Here's how the part is built. I have some questions about the finished solid (model axes, mm). Face numbers are marked on the shaded views. A direction names the side the tool comes from. Round coordinates to 2 decimals unless told otherwise and drop trailing zeros. Order: outer loops, then holes, each group sorted by start corner. A loop starts at its lowest first (then second) coordinate and runs counter-clockwise, first axis right, second up.
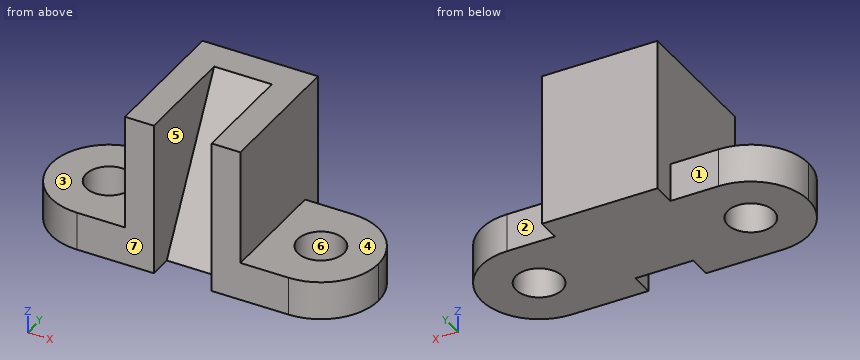
```python
from build123d import *

# Parameters (mm, degrees)
EXTRUDE_1_DEPTH     = 10
SKETCH_3_W          = 30
SKETCH_3_H          = 36
EXTRUDE_2_DEPTH     = 30
SKETCH_4_R          = 6
CUT_EXTRUDE_1_DEPTH = 52
CUT_EXTRUDE_START   = -7.5
CUT_EXTRUDE_2_DEPTH = 15


with BuildPart() as part:
    # 草图1 → 凸台-拉伸1 (new body)
    with BuildSketch(Plane.XY):
        with BuildLine():
            Line((15, -18), (-15, -18))
            Line((-15, -18), (-27.5, -18))
            ThreePointArc((-27.5, -18), (-38.106601718, -13.606601718), (-42.5, -3))
            ThreePointArc((-42.5, -3), (-38.106601718, 7.606601718), (-27.5, 12))
            Line((-27.5, 12), (-15, 12))
            Line((-15, 12), (-15, 18))
            Line((-15, 18), (15, 18))
            Line((15, 18), (15, 12))
            Line((15, 12), (27.5, 12))
            ThreePointArc((27.5, 12), (38.106601718, 7.606601718), (42.5, -3))
            ThreePointArc((42.5, -3), (38.106601718, -13.606601718), (27.5, -18))
            Line((27.5, -18), (15, -18))
        make_face()
    extrude(amount=EXTRUDE_1_DEPTH)

    # 草图3 → 凸台-拉伸2 (add)
    with BuildSketch(Plane.XY.offset(10)):
        Rectangle(SKETCH_3_W, SKETCH_3_H)
    extrude(amount=EXTRUDE_2_DEPTH)

    # 草图4 → 切除-拉伸1 (cut)
    with BuildSketch(Plane.XY):
        with Locations(Location((-27.5, -3, 0), (0, 0, 180))):
            Circle(SKETCH_4_R)
        with Locations(Location((27.511001478, -3, 0), (0, 0, 180))):
            Circle(SKETCH_4_R)
    extrude(amount=CUT_EXTRUDE_1_DEPTH, mode=Mode.SUBTRACT)

    # 草图5 → 切除-拉伸2 (cut)
    with BuildSketch(Plane.ZY.offset(15).offset(CUT_EXTRUDE_START)):
        Polygon((40, 10), (0, -12), (0, -18), (40, -18), align=None)
    extrude(amount=-CUT_EXTRUDE_2_DEPTH, mode=Mode.SUBTRACT)


solid = part.part
```
1. If we section it at D-D, the plane z = 28: Write out the boundary of the cut face in (x, y), and give its area (3 significant figures).
Evaluation:
outline: (-15, -18) - (-7.5, -18) - (-7.5, 3.4) - (7.5, 3.4) - (7.5, -18) - (15, -18) - (15, 18) - (-15, 18) - close
area: 759 mm2
2. If we section it at C-C, the plane z = 3: Write out the boundary of the cut face in (x, y), and give its area (3 significant figures).
Evaluation:
outline: (-27.5, -18) - (-7.5, -18) - (-7.5, -10.35) - (7.5, -10.35) - (7.5, -18) - (27.5, -18) arc R15 ccw to (27.5, 12) - (15, 12) - (15, 18) - (-15, 18) - (-15, 12) - (-27.5, 12) arc R15 ccw to start; hole circle Ø12 at (-27.5, -3); hole circle Ø12 at (27.51, -3)
area: 2,200 mm2
3. I'm going to push flat-ended pins straight in: P1, Ø12, axis at y = 12, z = 26, coming from the +X side; P2, Ø8.5, axis at y = 1, z = 20.5, coming from the -X side; P3, Ø11, axis at x = -21, z = 5, coming from the +Y side. Where does each tip first touch, or does it pass through?
Evaluation:
P1: stops at x = 15
P2: stops at x = -15
P3: stops at y = 12
4. If we section it at A-A, the plane y = -15: Write out the boundary of the cut face in (x, z), and give its area (3 significant figures).
Evaluation:
outline: (-36.5, 0) - (-7.5, 0) - (-7.5, 40) - (-15, 40) - (-15, 10) - (-36.5, 10) - close; (7.5, 0) - (36.5, 0) - (36.5, 10) - (15, 10) - (15, 40) - (7.5, 40) - close
area: 1,030 mm2
5. I need wall thicknesses on probe 1 along Y at (x, z) = (-27.5, 2.25); probe 2 along X at (y, z) = (2, 38); probe 3 along Z at (x, y) = (36, -2). Which ranges of each line are inside material? Lowest first, please.
Evaluation:
probe 1: y = -18 to -9, 3 to 12
probe 2: x = -15 to -7.5, 7.5 to 15
probe 3: z = 0 to 10
6. If we section it at B-B, the plane y = 1: Write out the boundary of the cut face in (x, z).
Evaluation:
outline: (-41.96, 0) - (-31.97, 0) - (-31.97, 10) - (-41.96, 10) - close; (-23.03, 0) - (23.04, 0) - (23.04, 10) - (15, 10) - (15, 40) - (7.5, 40) - (7.5, 23.64) - (-7.5, 23.64) - (-7.5, 40) - (-15, 40) - (-15, 10) - (-23.03, 10) - close; (31.98, 0) - (41.96, 0) - (41.96, 10) - (31.98, 10) - close
7. If we mould it in two halves opening along X, with no side actions, what happens to the marked faces 6 and 7? For each: released by +X, released by -X, zero draft, split by the parting line, or undercut.
Evaluation:
face 6: undercut
face 7: zero draft
8. On a 3-axis mill with a long thin cutter (end or side, diameter ignored), from which of +Z, -Z, +X, -X, +Y, -Y can I reach the whole of each face in a straight line? I mean the marked faces 1, 2, 3, 4 and 5. Say none if no direction works.
Evaluation:
face 1: +Z, -Z, -X, +Y
face 2: +Z, -Z, +X, +Y
face 3: +Z, -X, +Y, -Y
face 4: +Z, +X, +Y, -Y
face 5: +Z, -Y
